Autodesk Inventor part; units mm, degrees
ref_plane "Work Plane1" through (1.525, 0, 0) normal (0, 0, 1) x (1, 0, 0)
ref_plane "YZ Plane" through (0, 0, 0) normal (1, 0, 0) x (0, 1, 0)
ref_plane "XZ Plane" through (0, 0, 0) normal (0, 1, 0) x (-1, 0, 0)
sketch "Sketch1" plane through (0, 0, 0) normal (0, 0, 1) x (1, 0, 0)
  line L0 (0, 7.1374) -> (0, 4.9276)
  line L1 (12.7, 4.7625) -> (127, 4.7625)
  line L2 (127, 4.7625) -> (127, 0)
  line L3 (127, 0) -> (-0.0001, 0)
  line L4 (-25.4001, 0) -> (152.4, 0)
  line L5 (-0.0001, 0) -> (-0.0001, 7.1374)
  line L6 (-0.0001, 7.1374) -> (0, 7.1374)
  line L7 (12.7, 4.7625) -> (8.7311, 4.9276)
  line L8 (8.7311, 4.9276) -> (0, 4.9276)
  line L9 (0, -1.4275) -> (0, 8.5649)
  dimension "d0" = 127
  dimension "d1" = 114.3
revolve "Body" add sketch "Sketch1" angle 360 about axis through (127, 0, 0) along (-1, 0, 0)
sketch "Sketch2" plane through (-0.0001, 0, 0) normal (-1, 0, 0) x (0, 0, 1)
  line L0 (0, 8.2416) -> (7.1374, 4.1208)
  line L1 (7.1374, 4.1208) -> (7.1374, -4.1208)
  line L2 (7.1374, -4.1208) -> (0, -8.2416)
  line L3 (0, -8.2416) -> (-7.1374, -4.1208)
  line L4 (-7.1374, -4.1208) -> (-7.1374, 4.1208)
  line L5 (-7.1374, 4.1208) -> (0, 8.2416)
  point P0 (0, 0)
  point P1 (0, 0)
  dimension "d11" = 14.2748
extrude "Head" add sketch "Sketch2" along normal blind 6.8072
sketch "Sketch4" plane through (0, 0, 0) normal (0, 0, 1) x (1, 0, 0)
  line L0 (-6.8073, 7.1374) -> (-6.8073, 8.2416)
  line L1 (-6.8073, 8.2416) -> (-6.1698, 8.2416)
  line L2 (-6.1698, 8.2416) -> (-6.8073, 7.1374)
  line L3 (-8.1687, 0) -> (1.3613, 0)
  line L4 (-0.0001, 8.2416) -> (-6.8073, 8.2416)
  line L5 (-6.8073, 4.1208) -> (-6.8073, 8.2416)
  dimension "d5" = 30
  dimension "d19" = 14.2748
revolve "Chamfer1" cut sketch "Sketch4" angle 360 about axis through (-10, 0, 0) along (1, 0, 0)
thread "Thread"
chamfer "Chamfer2" distance 0.9739 distance2 0.9447 1 edges at (127, -4.7625, 0) measured on face at (127, -0.1914, -0.5295)
ref_plane "Work Plane1" through (1.525, 0, 0) normal (0, 0, 1) x (1, 0, 0)
fillet "Fillet2" radius 0.762 1 edges at (0, -4.9276, 0)
equation "\"d11\" = SW"
equation "\"d3\" = KOH - SD"
equation "\"d63\" = R"
equation "\"d15\" = GEL"
equation "\"d6\" = -0.5 * SPD + 0.5 * GD"
equation "\"d5\" = ANG1"
equation "\"d19\" = SW0"
equation "\"NLG\" = 190.5"
equation "\"GD\" = NND"
equation "\"BDM\" = 9.8552"
equation "\"KOH\" = 6.8072"
equation "\"GEL\" = 31.75"
equation "\"SW\" = 14.2748"
equation "\"SW0\" = SW"
equation "\"SPD\" = GD1"
equation "\"SD2\" = SW"
equation "\"SD\" = 0"
equation "\"ANG1\" = 30deg"
equation "\"GAL\" = 3.96875"
equation "\"GUL\" = 0.238 * GAL"
equation "\"R\" = 0.762"
equation "\"d62\" = -NLG - SD + GUL"
equation "\"GD1\" = 7.5773"
equation "\"THREADDIA\" = 9.525"
equation "\"TOA\" = 30deg"
equation "\"NND\" = 9.525"
equation "\"E0\" = 1.155 * SW"
properties part number "am-1055" material "Steel, Mild"
Geometry check sheet. Reference: the model listing, model coordinates, mm. A direction names the side the tool comes from. Coordinates: 2 decimals unless noted, no trailing zeros. Write each loop counter-clockwise with the first axis right and the second up, starting at its lowest first coordinate (ties: lowest second). Pieces come first, ordered by that corner, then holes. Notation, with made-up numbers: M 41,-33.5 L 100,-33.5 A6 cw 100,-26.5 Z; hole C 1,36.25 d9. An arc over 180 degrees is marked long. Answer as a JSON object with one key per item and string values.
1. Go/stop test with flat-tipped pins: pin 1 Ø4 at (x, y) = (103, 1) entering from -Z; pin 2 Ø3 at (x, z) = (97, 0.5) entering from +Y; pin 3 Ø2 at (x, z) = (50, -5) entering from +Y. Record where each tip stops, or that it passes through.
Answers below:
{"pin 1": "stops at z = -4.76", "pin 2": "stops at y = 4.76", "pin 3": "stops at y = 2.58"}
2. Section check A-A, the plane x = 109.5. Enter the section's corners in (y, z) (1 decimal), plus the area to 3 significant figures.
Answers below:
{"outline": "C 0,0 d9.5", "area": "71.3 mm²"}
3. Scan lines: L1, parallel to X at y = 3.25, z = 6; L2, parallel to Z at x = 47.5, y = -0.25; L3, parallel to Y at x = 14, z = -0.5. Record each from-to range of solid material in increasing order.
Answers below:
{"L1": "x = -6.81 to 0", "L2": "z = -4.76 to 4.76", "L3": "y = -4.74 to 4.74"}
4. Tool access check on faces 1 (the flat face through (-6.807, 0, 0)), 2 (the cylindrical face through (4.691, -4.923, -0.217)). Record the directions out of +Z, -Z, +X, -X, +Y, -Y that give a thin tool (end or side, any length) a straight path to the whole face; none if there is none.
Answers below:
{"face 1": "+Z, -Z, -X, +Y, -Y", "face 2": "+X"}
